```python
from build123d import *

# Parameters (mm, degrees)
SKETCH1_W           = 56
SKETCH1_H           = 35
SKETCH1_R           = 1.2
BOSS_EXTRUDE1_DEPTH = 38.4
SKETCH2_R           = 3
SKETCH2_R_2         = 1.2
BOSS_EXTRUDE2_DEPTH = 3.6
FILLET2_R           = 3


with BuildPart() as part:
    # Sketch1 → Boss-Extrude1 (new body)
    with BuildSketch(Plane(origin=(0, 0, 0), x_dir=(1, 0, 0), z_dir=(0, 1, 0))):
        Rectangle(SKETCH1_W, SKETCH1_H)
        with Locations(Location((-22.38, 14, 0), (0, 0, 270))):
            Circle(SKETCH1_R, mode=Mode.SUBTRACT)
        with Locations(Location((4.62, 14, 0), (0, 0, 270))):
            Circle(SKETCH1_R, mode=Mode.SUBTRACT)
        with Locations(Location((-22.38, -14, 0), (0, 0, 270))):
            Circle(SKETCH1_R, mode=Mode.SUBTRACT)
        with Locations(Location((4.62, -14, 0), (0, 0, 270))):
            Circle(SKETCH1_R, mode=Mode.SUBTRACT)
        with Locations(Location((23.52, 13.5, 0), (0, 0, 270))):
            Circle(SKETCH1_R, mode=Mode.SUBTRACT)
        with Locations(Location((23.52, -13.5, 0), (0, 0, 270))):
            Circle(SKETCH1_R, mode=Mode.SUBTRACT)
    extrude(amount=BOSS_EXTRUDE1_DEPTH)

    # Sketch2 → Boss-Extrude2 (add)
    with BuildSketch(Plane.XZ):
        with Locations(Location((-15.38, 0, 0), (0, 0, 90))):
            Circle(SKETCH2_R)
        with Locations(Location((-15.38, 0, 0), (0, 0, 270))):
            Circle(SKETCH2_R_2, mode=Mode.SUBTRACT)
    boss_extrude2 = extrude(amount=BOSS_EXTRUDE2_DEPTH)

    # Mirror2: Boss-Extrude2 across plane
    add(boss_extrude2.mirror(Plane(origin=(0, 19.2, 0), x_dir=(0, 0, 1), z_dir=(0, -1, 0))))

    # Fillet2
    fillet2_edges = [part.edges().sort_by_distance(p)[0] for p in [
        (-15.38, 0, -3),
        (-15.38, 38.4, -3),
        (-28, 19.2, -17.5),
        (28, 19.2, -17.5),
        (28, 19.2, 17.5),
        (-28, 19.2, 17.5),
    ]]
    fillet(fillet2_edges, radius=FILLET2_R)


solid = part.part
```
Part model, mm, in its own coordinate system. A direction names the side the tool comes from. Round coordinates to 2 decimals unless told otherwise and drop trailing zeros. Write each loop counter-clockwise with the first axis right and the second up, starting at its lowest first coordinate (ties: lowest second). Pieces come first, ordered by that corner, then holes. Notation, with made-up numbers: M 3,-19.75 L 15,-19.75 A14 cw 15,-10.75 Z; hole C 8.25,-22.5 d6. An arc over 180 degrees is marked long. Answer as CSV lines item,"result". Start each with the question number.
1) Band-saw the part on A-A (x = 23.52). List the corners of the cut face in (y, z), then the cut area to 3 significant figures.
2) Drop flat-ended pins along their axis: pin 1 (4 mm diameter, centred on x = -22.38, z = 14, fed in from -Y); pin 2 (3 mm diameter, centred on x = 23.52, z = 13.5, fed in from +Y). Give the stop position or say it passes through.
3) Band-saw the part on C-C (z = 13.5). List the corners of the cut face in (x, y), then the cut area to 3 significant figures.
4) Which spindle directions (+Z, -Z, +X, -X, +Y, -Y) get a long thin tool onto all of the face, cutting with end or side? Do faces 4 (the face through (-15, 0, 0)), 5 (the face through (-12.45, 41.7, -0.65)), 6 (the face through (5.431, 18.931, 13.116)). Say none if no direction does.
5) Drill centre lines: L1, parallel to Z at x = -22.5, y = 29; L2, parallel to Z at x = 22.5, y = 6.5; L3, parallel to X at y = 15, z = -13. Where is each one in solid material? Low to high.
6) Band-saw the part on D-D (x = -15.38). List the corners of the cut face in (y, z).
7) Band-saw the part on B-B (y = 2). List the corners of the cut face in (x, z).
8) Mould opens along X. For faces 1 (the face through (22.35, 18.93, 13.24)), 2 (the face through (0, 0, 0)), 3 (the face through (28, 19, 0)) say: +X half, -X half, draft (parallel to the pull), parting line (faces both ways), or undercut.
Worked out:
1,outline,"M 0,-17.5 L 38.4,-17.5 L 38.4,-14.7 L 0,-14.7 Z; M 0,-12.3 L 38.4,-12.3 L 38.4,12.3 L 0,12.3 Z; M 0,14.7 L 38.4,14.7 L 38.4,17.5 L 0,17.5 Z"
1,area,"1,160 mm²"
2,pin 1,"y = 0"
2,pin 2,"y = 38.4"
3,outline,"M -28,0 L -23.47,0 L -23.47,38.4 L -28,38.4 Z; M -21.29,0 L 3.53,0 L 3.53,38.4 L -21.29,38.4 Z; M 5.71,0 L 22.32,0 L 22.32,38.4 L 5.71,38.4 Z; M 24.72,0 L 28,0 L 28,38.4 L 24.72,38.4 Z"
3,area,"1,890 mm²"
4,face 4,"-Y"
4,face 5,"+Y"
4,face 6,"+Y, -Y"
5,L1,"-17.5 to -15.19, -12.81 to 12.81, 15.19 to 17.5"
5,L2,"-17.5 to -14.13, -12.87 to 12.87, 14.13 to 17.5"
5,L3,"-28 to -23.04, -21.72 to 3.96, 5.28 to 22.43, 24.61 to 28"
6,outline,"M -3.6,-3 L -3,-3 A3 cw 0,-6 L 0,-17.5 L 38.4,-17.5 L 38.4,-6 A3 cw 41.4,-3 L 42,-3 L 42,-1.2 L 38.4,-1.2 L 38.4,1.2 L 42,1.2 L 42,3 L 41.4,3 A3 cw 38.4,6 L 38.4,17.5 L 0,17.5 L 0,6 A3 cw -3,3 L -3.6,3 L -3.6,1.2 L 0,1.2 L 0,-1.2 L -3.6,-1.2 Z"
7,outline,"M -28,-14.5 A3 ccw -25,-17.5 L 25,-17.5 A3 ccw 28,-14.5 L 28,14.5 A3 ccw 25,17.5 L -25,17.5 A3 ccw -28,14.5 Z; hole C -22.38,-14 d2.4; hole C -22.38,14 d2.4; hole C 4.62,-14 d2.4; hole C 4.62,14 d2.4; hole C 23.52,-13.5 d2.4; hole C 23.52,13.5 d2.4"
8,face 1,"undercut"
8,face 2,"draft"
8,face 3,"+X half"
